```python
from build123d import *

# Parameters (mm, degrees)
F0_R     = 25
F0_R_2   = 7.9354206637
F1_DEPTH = 0.7
F0_R_3   = 4.15
F2_DEPTH = 1.7
F3_DEPTH = 4


# Not quite as in the source:
# - a fillet or chamfer that OpenCascade refuses, or shapes differently, is made with other operations: its cross-section is extruded or revolved along the edge and cut away or added


with BuildPart() as f1:
    # F0 (on Top) → F1 (new body)
    with BuildSketch(Plane.XY):
        Circle(F0_R)
        Circle(F0_R_2, mode=Mode.SUBTRACT)
    extrude(amount=F1_DEPTH)

    # F0 (on Top) → F2 (join)
    with BuildSketch(Plane.XY):
        Circle(F0_R_2)
        Circle(F0_R_3, mode=Mode.SUBTRACT)
    extrude(amount=F2_DEPTH)

    # F0 (on Top) → F3 (join)
    with BuildSketch(Plane.XY):
        Circle(F0_R_3)
    extrude(amount=F3_DEPTH)

    # F4: chamfer of 2 on 1 edges, made by hand

    # F4_s1 → F4_t2 (revolve, cut)
    with BuildSketch(Plane.XZ):
        Polygon((25, 2), (23, 0), (25, 0), align=None)
    revolve(axis=Axis((0, 0, 0), (0, 0, 1)), mode=Mode.SUBTRACT)


solid = f1.part
```
Model file for the job. Use its own axes, mm. A direction names the side the tool comes from. Give positions to 0.01 mm unless a question says otherwise; leave off trailing zeros. Loops run counter-clockwise (first coordinate to the right, second up) from the corner with the lowest first, then second, coordinate; pieces in that order, holes last. Notation, with made-up numbers: (1.5, 0) -> (5.5, 0) arc R18 cw to (5.5, 6) -> close; hole circle Ø10 at (40.5, 28.25). An arc over 180 degrees is marked (long way). Write each question's results on one line, items separated by ' | '.
(1) Flat gauge pin, fed straight in: pin 1 Ø12 at (x, y) = (16, -12.5) entering from +Z. Where does the tip first touch, or does it go through?
Geometry results:
pin 1: stops at z = 0.7
(2) Probe line 1 along Z through (x, y) = (7.5, -7.5); line 2 along Z through (x, y) = (-6, -1); line 3 along Y through (x, z) = (2, 2.75). List the from-to ranges inside material, lowest first.
Geometry results:
line 1: z = 0 to 0.7 | line 2: z = 0 to 1.7 | line 3: y = -3.64 to 3.64
(3) Tool access for faces 1 (the cylindrical face through (-6.297, -4.829, 1.193)), 2 (the flat face through (0, 0, 4)): list every direction of +Z, -Z, +X, -X, +Y, -Y with a clear straight run to the whole face (end or side of a thin tool).
Geometry results:
face 1: +Z | face 2: +Z, +X, -X, +Y, -Y
(4) Cut at C-C on z = 2.9. List the corners of the cut face in (x, y), and give its area (3 significant figures).
Geometry results:
outline: circle Ø8.3 at (0, 0) | area: 54.1 mm²
(5) Cut at A-A on y = 0. List the corners of the cut face in (x, z), and give its area (3 significant figures).
Geometry results:
outline: (-23.7, 0.7) -> (-23, 0) -> (23, 0) -> (23.7, 0.7) -> (7.94, 0.7) -> (7.94, 1.7) -> (4.15, 1.7) -> (4.15, 4) -> (-4.15, 4) -> (-4.15, 1.7) -> (-7.94, 1.7) -> (-7.94, 0.7) -> close | area: 67.7 mm²
